Work out the finished part from the listing and answer in its coordinate system (mm). A direction names the side the tool comes from. Give positions to 0.01 mm unless a question says otherwise; leave off trailing zeros. Write each loop counter-clockwise with the first axis right and the second up, starting at its lowest first coordinate (ties: lowest second). Pieces come first, ordered by that corner, then holes. Notation, with made-up numbers: (43.5, -16.5) -> (69.5, -16.5) arc R35 ccw to (69.5, 15.5) -> close; hole circle Ø8 at (42.25, 3.25). An arc over 180 degrees is marked (long way). Write item = value, one per line. Start each with the question number.
from build123d import *

# Parameters (mm, degrees)
BOSS_EXTRUDE2_DEPTH      = 6
BOSS_EXTRUDE2_DEPTH_BACK = 6
SKETCH1_W                = 180
SKETCH1_H                = 50
SKETCH3_R                = 3.5
BOSS_EXTRUDE3_DEPTH      = 6


with BuildPart() as part:
    # Sketch1 → Boss-Extrude2 (new, two sides: drawn at the far end of the back side and taken through both)
    with BuildSketch(Plane.XY.offset(-BOSS_EXTRUDE2_DEPTH_BACK)):
        Rectangle(SKETCH1_W, SKETCH1_H)
    extrude(amount=BOSS_EXTRUDE2_DEPTH + BOSS_EXTRUDE2_DEPTH_BACK)

    # Sketch3 → Boss-Extrude3 (add)
    with BuildSketch(Plane.XZ.offset(25)):
        with Locations(Location((84, 0, 0), (0, 0, 270))):
            Circle(SKETCH3_R)
    extrude(amount=BOSS_EXTRUDE3_DEPTH)


solid = part.part
(1) A cutting plane is placed at D-D, the plane x = -12. Write down the section's boundary in (y, z), then the cut area to 3 significant figures.
(2) A cutting plane is placed at A-A, the plane x = 84. Write down the section's boundary in (y, z), then the cut area to 3 significant figures.
(3) For faces 1 (the cylindrical face through (80.583, -27.958, 0.759)), 2 (the flat face through (-90, 0, 0)), determine the directions among +Z, -Z, +X, -X, +Y, -Y from which every point of the face is accessible in a straight line to the end or side of a thin tool.
(4) A cutting plane is placed at B-B, the plane z = 0. Write down the section's boundary in (x, y).
(5) A cutting plane is placed at C-C, the plane y = -27. Write down the section's boundary in (x, z), then the cut area to 3 significant figures.
(6) Find the intervals of material crossed by line 1 along Y through (x, z) = (5.5, -5), in increasing order.
(7) This flat-tipped pin is pushed along its axis until it touches: pin 1 (4 mm diameter, centred on x = -44, z = -1, fed in from -Y). Where does it stop, or does it pass through?
Results list:
q1.outline = (-25, -6) -> (25, -6) -> (25, 6) -> (-25, 6) -> close
q1.area = 600 mm²
q2.outline = (-31, -3.5) -> (-25, -3.5) -> (-25, -6) -> (25, -6) -> (25, 6) -> (-25, 6) -> (-25, 3.5) -> (-31, 3.5) -> close
q2.area = 642 mm²
q3.face_1 = -Y
q3.face_2 = +Z, -Z, -X, +Y, -Y
q4.outline = (-90, -25) -> (80.5, -25) -> (80.5, -31) -> (87.5, -31) -> (87.5, -25) -> (90, -25) -> (90, 25) -> (-90, 25) -> close
q5.outline = circle Ø7 at (84, 0)
q5.area = 38.5 mm²
q6.line_1 = -25 to 25
q7.pin_1 = -25
